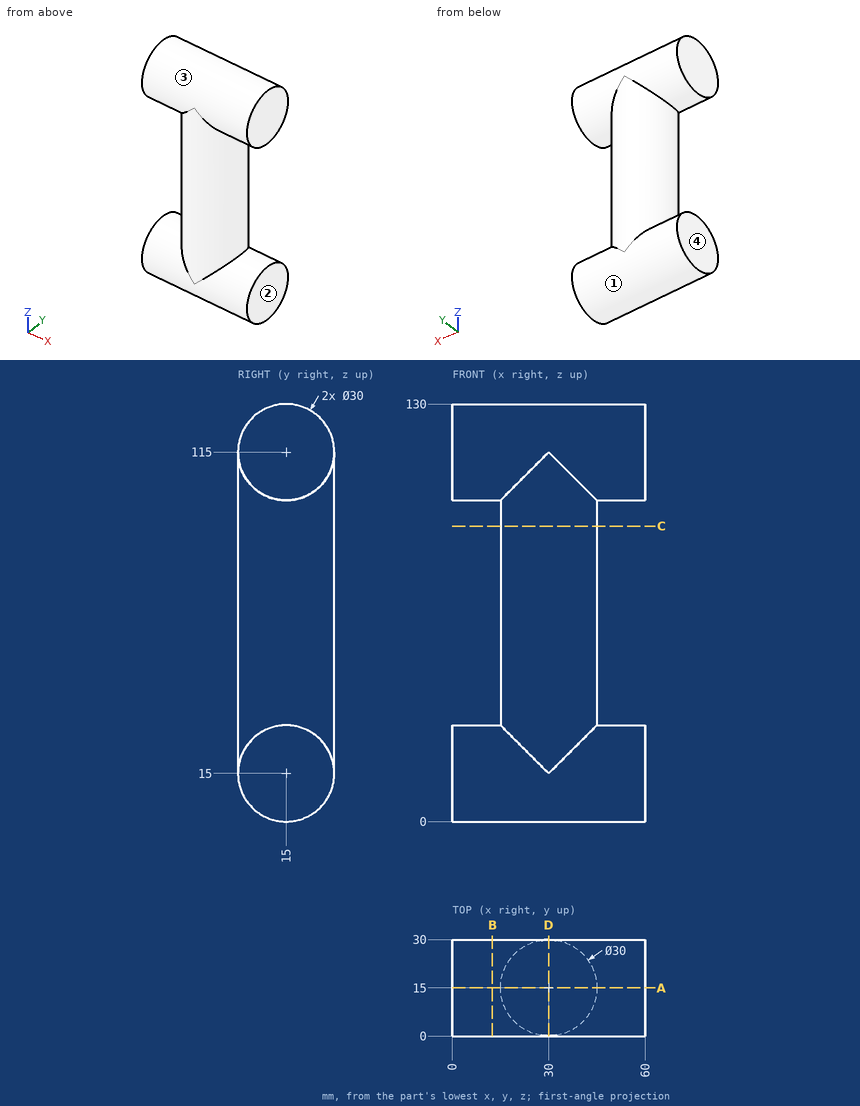
Study the drawing (mm; zero at the part's minimum x, y, z) and answer. A direction names the side the tool comes from. Give positions to 0.01 mm unless a question says otherwise; leave off trailing zeros. Order: outer loops, then holes, each group sorted by start corner. A loop starts at its lowest first (then second) coordinate and runs counter-clockwise, first axis right, second up. Notation, with made-up numbers: (3.25, 44.25) - (19.25, 44.25) arc R29 cw to (19.25, 70.25) - close; hole circle Ø9 at (18, -15.75). An arc over 180 degrees is marked (long way). Answer as CSV lines item,"result". Start each with the question number.
Q1. The part is cut by section D-D (x = 30). Write down the section's boundary in (y, z).
Q2. The part is cut by section C-C (z = 92). Write down the section's boundary in (x, y).
Q3. The part is cut by section B-B (x = 12.5). Write down the section's boundary in (y, z), then the cut area to 3 significant figures.
Q4. The mould has two halves that part along Z. Classify the marked faces 1 and 2: +Z half, -Z half, draft (parallel to the pull), parting line (faces both ways), or undercut.
Q5. The part is cut by section A-A (y = 15). Write down the section's boundary in (x, z), then the cut area to 3 significant figures.
Q6. For the marked faces 3 and 4, determine the directions among +Z, -Z, +X, -X, +Y, -Y from which every point of the face is accessible in a straight line to the end or side of a thin tool.
Q7. Find the intervals of material crossed by L1, parallel to Z at x = 9, y = 4.75; L2, parallel to Z at x = 15, y = 10.75; L3, parallel to Y at x = 12, z = 110, in increasing order. Write a range as [from, to].
Q8. Given pin 1 Ø1.5 at (x, z) = (16.5, 87.5) entering from -Y; pin 2 Ø4 at (x, y) = (51, 9) entering from -Z; pin 3 Ø10 at (x, y) = (21, 21.5) entering from -Z, each flat-ended and moving along its own axis, determine where each tip first touches the part or whether it passes through.
Check result:
1,outline,"(0, 15) arc R15 ccw to (30, 15) - (30, 115) arc R15 ccw to (0, 115) - close"
2,outline,"circle Ø30 at (30, 15)"
3,outline,"circle Ø30 at (15, 15); circle Ø30 at (15, 115)"
3,area,"1,410 mm²"
4,face 1,"undercut"
4,face 2,"draft"
5,outline,"(0, 0) - (60, 0) - (60, 30) - (45, 30) - (45, 100) - (60, 100) - (60, 130) - (0, 130) - (0, 100) - (15, 100) - (15, 30) - (0, 30) - close"
5,area,"5,700 mm²"
6,face 3,"none"
6,face 4,"+Z, -Z, -X, +Y, -Y"
7,L1,"z = [4.05, 25.95], [104.05, 125.95]"
7,L2,"z = [0.61, 29.39], [100.61, 129.39]"
7,L3,"y = [0.86, 29.14]"
8,pin 1,"stops at y = 7.1"
8,pin 2,"stops at z = 0.54"
8,pin 3,"stops at z = 0.08"
